```python
from build123d import *

# Parameters (mm, degrees)
F1_DEPTH = 3
F2_SIZE2 = 4
F2_SIZE  = 2.2
F3_R     = 2.5
F5_DEPTH = 1
F6_R     = 0.4


with BuildPart() as f1:
    # F0 (on Top) → F1 (new body)
    with BuildSketch(Plane.XY):
        with BuildLine():
            Line((84, 6), (84, 51))
            Line((84, 51), (0, 51))
            Line((0, 51), (0, 45))
            ThreePointArc((0, 45), (4.070965, 26.5), (0, 8))
            Line((0, 8), (0, 6))
            Line((0, 6), (3.5, 0))
            Line((3.5, 0), (6, 6))
            Line((6, 6), (9.5, 0))
            Line((9.5, 0), (12, 6))
            Line((12, 6), (15.5, 0))
            Line((15.5, 0), (18, 6))
            Line((18, 6), (21.5, 0))
            Line((21.5, 0), (24, 6))
            Line((24, 6), (27.5, 0))
            Line((27.5, 0), (30, 6))
            Line((30, 6), (33.5, 0))
            Line((33.5, 0), (36, 6))
            Line((36, 6), (39.5, 0))
            Line((39.5, 0), (42, 6))
            Line((42, 6), (45.5, 0))
            Line((45.5, 0), (48, 6))
            Line((48, 6), (51.5, 0))
            Line((51.5, 0), (54, 6))
            Line((54, 6), (57.5, 0))
            Line((57.5, 0), (60, 6))
            Line((60, 6), (63.5, 0))
            Line((63.5, 0), (66, 6))
            Line((66, 6), (69.5, 0))
            Line((69.5, 0), (72, 6))
            Line((72, 6), (75.5, 0))
            Line((75.5, 0), (78, 6))
            Line((78, 6), (81.5, 0))
            Line((81.5, 0), (84, 6))
        make_face()
    extrude(amount=F1_DEPTH)

    # F2
    f2_edges = [f1.edges().sort_by_distance(p)[0] for p in [
        (0, 7, 3),
        (4.070965, 26.5, 3),
        (42, 51, 3),
        (0, 48, 3),
    ]]
    chamfer(f2_edges, length=F2_SIZE, length2=F2_SIZE2)

    # F3
    f3_edges = [f1.edges().sort_by_distance(p)[0] for p in [
        (0, 51, 0.4),
        (84, 51, 0.4),
    ]]
    fillet(f3_edges, radius=F3_R)

    # F4 (on face) → F5 (cut)
    with BuildSketch(Plane.XY.offset(3)):
        with BuildLine():
            Line((81.185907, 4.706178), (81.9, 6.42))
            Line((81.9, 6.42), (81.9, 44.9))
            Line((81.9, 44.9), (6.675109, 44.9))
            ThreePointArc((6.675109, 44.9), (10.170108, 26.793334), (6.887072, 8.647038))
            Line((6.887072, 8.647038), (9.185907, 4.706178))
            Line((9.185907, 4.706178), (11.685907, 10.706178))
            Line((11.685907, 10.706178), (15.185907, 4.706178))
            Line((15.185907, 4.706178), (17.685907, 10.706178))
            Line((17.685907, 10.706178), (21.185907, 4.706178))
            Line((21.185907, 4.706178), (23.685907, 10.706178))
            Line((23.685907, 10.706178), (27.185907, 4.706178))
            Line((27.185907, 4.706178), (29.685907, 10.706178))
            Line((29.685907, 10.706178), (33.185907, 4.706178))
            Line((33.185907, 4.706178), (35.685907, 10.706178))
            Line((35.685907, 10.706178), (39.185907, 4.706178))
            Line((39.185907, 4.706178), (41.685907, 10.706178))
            Line((41.685907, 10.706178), (45.185907, 4.706178))
            Line((45.185907, 4.706178), (47.685907, 10.706178))
            Line((47.685907, 10.706178), (51.185907, 4.706178))
            Line((51.185907, 4.706178), (53.685907, 10.706178))
            Line((53.685907, 10.706178), (57.185907, 4.706178))
            Line((57.185907, 4.706178), (59.685907, 10.706178))
            Line((59.685907, 10.706178), (63.185907, 4.706178))
            Line((63.185907, 4.706178), (65.685907, 10.706178))
            Line((65.685907, 10.706178), (69.185907, 4.706178))
            Line((69.185907, 4.706178), (71.685907, 10.706178))
            Line((71.685907, 10.706178), (75.185907, 4.706178))
            Line((75.185907, 4.706178), (77.685907, 10.706178))
            Line((77.685907, 10.706178), (81.185907, 4.706178))
        make_face()
    extrude(amount=-F5_DEPTH, mode=Mode.SUBTRACT)

    # F6
    f6_edges = [f1.edges().sort_by_distance(p)[0] for p in [
        (84, 27.25, 0),
        (83.267767, 50.267767, 0),
        (82.75, 3, 0),
        (42, 51, 0),
        (79.75, 3, 0),
        (0.732233, 50.267767, 0),
        (76.75, 3, 0),
        (0, 46.75, 0),
        (73.75, 3, 0),
        (4.070965, 26.5, 0),
        (70.75, 3, 0),
        (0, 7, 0),
        (67.75, 3, 0),
        (1.75, 3, 0),
        (64.75, 3, 0),
        (4.75, 3, 0),
        (61.75, 3, 0),
        (7.75, 3, 0),
        (58.75, 3, 0),
        (10.75, 3, 0),
        (55.75, 3, 0),
        (13.75, 3, 0),
        (52.75, 3, 0),
        (16.75, 3, 0),
        (49.75, 3, 0),
        (19.75, 3, 0),
        (46.75, 3, 0),
        (22.75, 3, 0),
        (43.75, 3, 0),
        (25.75, 3, 0),
        (40.75, 3, 0),
        (28.75, 3, 0),
        (37.75, 3, 0),
        (31.75, 3, 0),
        (34.75, 3, 0),
    ]]
    fillet(f6_edges, radius=F6_R)


solid = f1.part
```
Source: CAD feature listing. Evaluate the final solid. Frame: model axes, mm. A direction names the side the tool comes from. Coordinates: 2 decimals unless noted, no trailing zeros. Return JSON: item names as keys, results as strings. Group by question number.
1) Contact query for flat-ended pins moving along their axis: P1, Ø6, axis at x = 69, y = 32, coming from the +Z side; P2, Ø1.1, axis at x = 48.5, z = 2.5, coming from the -Y side; P3, Ø1.5, axis at y = 27.5, z = 1, coming from the -X side. Output: stop coordinate, or through.
2) Set-up query: faces 1 (the face through (46.732, 2.958, 1.682)), 2 (the face through (4.813, 3.465, 0.114)), 3 (the face through (67.41, 7.75, 2.51)). Return all of +Z, -Z, +X, -X, +Y, -Y with unobstructed straight access to the full face (end or side cutting, diameter ignored); none if empty.
3) Mould query, pull axis X, two halves, no side actions, for faces 4 (the face through (82.732, 2.958, 1.682)), 5 (the face through (4.732, 2.958, 1.682)), 6 (the face through (2.47, 4.94, 2.16)). Classes: +X half, -X half, draft (parallel to the pull), parting line (faces both ways), or undercut.
4) Ray query, line 1 along Z through (x, y) = (34, 18); line 2 along X through (y, z) = (18.5, 2.55); line 3 along X through (y, z) = (39, 2.6). Return the intervals inside material, ascending.
From the geometry:
{
 "1": {"P1": "z = 2", "P2": "y = 4.2", "P3": "x = 4.04"},
 "2": {"face 1": "+Z, -Z, -Y", "face 2": "-Z, -Y", "face 3": "+Z"},
 "3": {"face 4": "+X half", "face 5": "undercut", "face 6": "-X half"},
 "4": {"line 1": "0 to 2", "line 2": "6.57 to 9.53, 81.9 to 84", "line 3": "5.66 to 8.59, 81.9 to 84"}
}
